from build123d import *

# Parameters (mm, degrees)
BOSS_EXTRUDE1_DEPTH = 10
SKETCH3_R           = 2
SKETCH3_R_2         = 20
CUT_EXTRUDE1_DEPTH  = 10


with BuildPart() as part:
    # Sketch2 → Boss-Extrude1 (new body)
    with BuildSketch(Plane.XY):
        with BuildLine():
            ThreePointArc((30, 41.243181255), (41.354060385, 29.846971198), (48.593569979, 15.481116133))
            add(Edge.make_bspline(
                [(30, 64.78657274), (30, 46.734360232), (43.458104798, 31.600792807), (48.593569979, 15.481116133)],
                knots=[0, 0, 0, 0, 1, 1, 1, 1], degree=3))
            Line((30, 64.78657274), (30, 41.243181255))
        make_face()
        with BuildLine():
            ThreePointArc((-48.593569979, 15.481116133), (-41.354060385, 29.846971198), (-30, 41.243181255))
            Line((-30, 41.243181255), (-30, 64.78657274))
            add(Edge.make_bspline(
                [(-30, 64.78657274), (-30, 46.734360232), (-43.458104798, 31.600792807), (-48.593569979, 15.481116133)],
                knots=[0, 0, 0, 0, 1, 1, 1, 1], degree=3))
        make_face()
        with BuildLine():
            add(Edge.make_bspline(
                [(-37.932636655, 137.306888623), (-30.736363595, 115.801238579), (-30, 113.598295334), (-30, 82.392834072)],
                knots=[0, 0, 0, 0, 1, 1, 1, 1], degree=3))
            Line((-30, 82.392834072), (-30, 123.542486889))
            ThreePointArc((-30, 123.542486889), (-34.65653574, 130.026904834), (-37.932636655, 137.306888623))
        make_face()
        with BuildLine():
            add(Edge.make_bspline(
                [(37.932636655, 137.306888623), (30.736363595, 115.801238579), (30, 113.598295334), (30, 82.392834072)],
                knots=[0, 0, 0, 0, 1, 1, 1, 1], degree=3))
            ThreePointArc((37.932636655, 137.306888623), (34.65653574, 130.026904834), (30, 123.542486889))
            Line((30, 123.542486889), (30, 82.392834072))
        make_face()
        with BuildLine():
            Line((30, 41.243181255), (30, 123.542486889))
            ThreePointArc((30, 123.542486889), (0, 190), (-30, 123.542486889))
            Line((-30, 123.542486889), (-30, 41.243181255))
            ThreePointArc((-30, 41.243181255), (-45.447772223, 23.140872931), (-51, 0))
            ThreePointArc((-51, 0), (0, -51), (51, 0))
            ThreePointArc((51, 0), (45.447772223, 23.140872931), (30, 41.243181255))
        make_face()
    extrude(amount=BOSS_EXTRUDE1_DEPTH)

    # Sketch3 → Cut-Extrude1 (cut)
    with BuildSketch(Plane.XY.offset(10)):
        with Locations((0, -47.5)):
            Circle(SKETCH3_R)
        with Locations((-47.5, 0)):
            Circle(SKETCH3_R)
        with Locations((0, 47.5)):
            Circle(SKETCH3_R)
        with Locations((47.5, 0)):
            Circle(SKETCH3_R)
        Circle(SKETCH3_R_2)
    extrude(amount=-CUT_EXTRUDE1_DEPTH, mode=Mode.SUBTRACT)


solid = part.part
Geometry check sheet. Reference: the model listing, model coordinates, mm. A direction names the side the tool comes from. Round coordinates to 2 decimals unless told otherwise and drop trailing zeros. Loops run counter-clockwise (first coordinate to the right, second up) from the corner with the lowest first, then second, coordinate; pieces in that order, holes last. Notation, with made-up numbers: (52, 12) -> (94, 12) arc R19 ccw to (94, 21) -> close; hole circle Ø4 at (12.25, 60). An arc over 180 degrees is marked (long way). Answer as a JSON object with one key per item and string values. Group by question number.
Item 1: Set-up check for faces 1 (the face through (-49.498, 0.088, 5.07)), 2 (the face through (-30, 74, 5)): record each of +Z, -Z, +X, -X, +Y, -Y from which the full face is reachable in a straight line by a thin tool's end or side.
Item 2: Cross-section at A-A, the plane x = 15. Record the cut outline in (y, z), plus the area to 3 significant figures.
Item 3: Cross-section at B-B, the plane y = 9. Record the cut outline in (x, z).
Item 4: Cross-section at C-C, the plane z = 7. Count the separate pieces of the cut face and the enclosed holes in it, plus the area to 3 significant figures.
Item 5: Depth check by flat-ended pin: pin 1 Ø6.5 at (x, y) = (-47.5, 0) entering from +Z; pin 2 Ø3 at (y, z) = (72.5, 5) entering from +X; pin 3 Ø3 at (x, y) = (47.5, 0) entering from -Z; pin 4 Ø5 at (y, z) = (12.5, 6) entering from +X. Enter the tip coordinate at first touch or a pass-through.
Item 6: Cross-section at D-D, the plane y = 150. Record the cut outline in (x, z).
Item 7: Release check for a two-part mould opening along X. For faces 3 (the face through (30, 73, 5)), 4 (the face through (-1, 71, 10)), 5 (the face through (-4.336, -19.524, 5.07)) record: pulls with the +X half, pulls with the -X half, needs draft (parallel to the pull), parting line crosses it, or undercut.
Item 8: Thickness scan on line 1 along Y through (x, z) = (0, 8.25); line 2 along X through (y, z) = (80.5, 1); line 3 along X through (y, z) = (47, 8.5). Record the ranges inside material, lowest first.
Determined:
{
 "1": {"face 1": "+Z, -Z", "face 2": "+Z, -Z, -X"},
 "2": {"outline": "(-48.74, 0) -> (-13.23, 0) -> (-13.23, 10) -> (-48.74, 10) -> close; (13.23, 0) -> (187.08, 0) -> (187.08, 10) -> (13.23, 10) -> close", "area": "2,090 mm²"},
 "3": {"outline": "(-50.2, 0) -> (-17.86, 0) -> (-17.86, 10) -> (-50.2, 10) -> close; (17.86, 0) -> (50.2, 0) -> (50.2, 10) -> (17.86, 10) -> close"},
 "4": {"separate pieces": "1", "enclosed holes": "5", "area": "16,100 mm²"},
 "5": {"pin 1": "stops at z = 10", "pin 2": "stops at x = 30", "pin 3": "passes through", "pin 4": "stops at x = 50.01"},
 "6": {"outline": "(-40, 0) -> (40, 0) -> (40, 10) -> (-40, 10) -> close"},
 "7": {"face 3": "pulls with the +X half", "face 4": "needs draft", "face 5": "undercut"},
 "8": {"line 1": "y = -51 to -49.5, -45.5 to -20, 20 to 45.5, 49.5 to 190", "line 2": "x = -30 to 30", "line 3": "x = -33.9 to -1.94, 1.94 to 33.9"}
}
